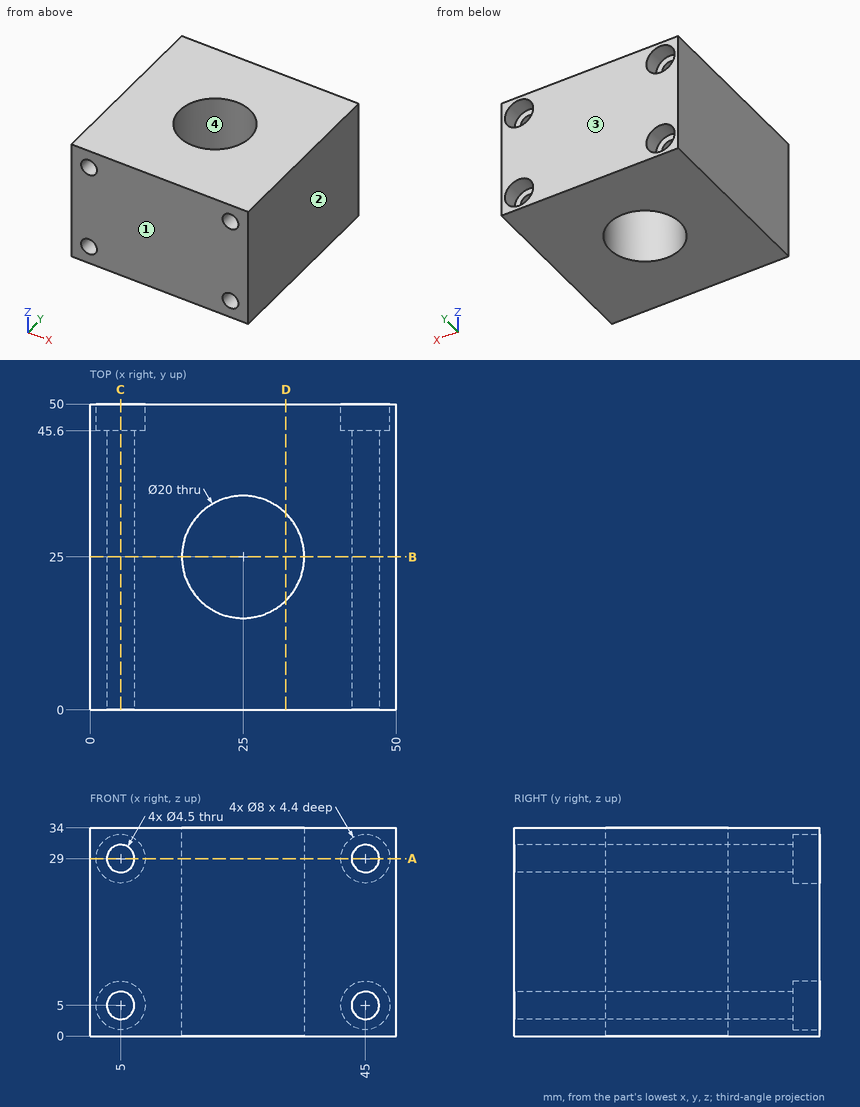
Job drawing, mm, ordinate dimensions from the low corner. One solid piece. Give positions to 0.01 mm unless a question says otherwise; leave off trailing zeros. Loops run counter-clockwise (first coordinate to the right, second up) from the corner with the lowest first, then second, coordinate; pieces in that order, holes last. Notation, with made-up numbers: M 45,-13 L 54,-13 A29 ccw 54,17 Z; hole C 20.25,74.5 d3. An arc over 180 degrees is marked long. Answer in a Markdown table with one row per item. Add a question column.
Item 1: Band-saw the part on A-A on z = 29. Give the cut face in (x, y).
Item 2: Mould opens along Y. For the marked faces 1, 2, 3 and 4 say: +Y half, -Y half, draft (parallel to the pull), parting line (faces both ways), or undercut.
Item 3: Band-saw the part on D-D on x = 32. Give the cut face in (y, z), then the cut area to 3 significant figures.
Item 4: Band-saw the part on B-B on y = 25. Give the cut face in (x, z).
Item 5: Probe probe 1 along Z at (x, y) = (5, 29); probe 2 along Z at (x, y) = (5, 48.4); probe 3 along X at (y, z) = (47, 29). List the from-to ranges inside material, lowest first.
Item 6: Drop flat-ended pins along their axis: P1, Ø5, axis at x = 45, z = 5, coming from the -Y side; P2, Ø4, axis at x = 4.5, z = 30.5, coming from the +Y side. Give the stop position or say it passes through.
Item 7: Band-saw the part on C-C on x = 5. Give the cut face in (y, z), then the cut area to 3 significant figures.
Reply:
| question | item | result |
|---|---|---|
| 1 | outline | M 0,0 L 2.75,0 L 2.75,45.6 L 1,45.6 L 1,50 L 0,50 Z; M 7.25,0 L 42.75,0 L 42.75,45.6 L 41,45.6 L 41,50 L 9,50 L 9,45.6 L 7.25,45.6 Z; M 47.25,0 L 50,0 L 50,50 L 49,50 L 49,45.6 L 47.25,45.6 Z; hole C 25,25 d20 |
| 2 | face 1 | -Y half |
| 2 | face 2 | draft |
| 2 | face 3 | +Y half |
| 2 | face 4 | undercut |
| 3 | outline | M 0,0 L 17.86,0 L 17.86,34 L 0,34 Z; M 32.14,0 L 50,0 L 50,34 L 32.14,34 Z |
| 3 | area | 1,210 mm^2 |
| 4 | outline | M 0,0 L 15,0 L 15,34 L 0,34 Z; M 35,0 L 50,0 L 50,34 L 35,34 Z; hole C 5,5 d4.5; hole C 5,29 d4.5; hole C 45,5 d4.5; hole C 45,29 d4.5 |
| 5 | probe 1 | z = 0 to 2.75, 7.25 to 26.75, 31.25 to 34 |
| 5 | probe 2 | z = 0 to 1, 9 to 25, 33 to 34 |
| 5 | probe 3 | x = 0 to 1, 9 to 41, 49 to 50 |
| 6 | P1 | stops at y = 0 |
| 6 | P2 | stops at y = 45.6 |
| 7 | outline | M 0,0 L 50,0 L 50,1 L 45.6,1 L 45.6,2.75 L 0,2.75 Z; M 0,7.25 L 45.6,7.25 L 45.6,9 L 50,9 L 50,25 L 45.6,25 L 45.6,26.75 L 0,26.75 Z; M 0,31.25 L 45.6,31.25 L 45.6,33 L 50,33 L 50,34 L 0,34 Z |
| 7 | area | 1,220 mm^2 |
